Check sheet for the modelled part. Datum: model origin and axes. Units: mm. Round coordinates to 2 decimals unless told otherwise and drop trailing zeros. Write each loop counter-clockwise with the first axis right and the second up, starting at its lowest first coordinate (ties: lowest second). Pieces come first, ordered by that corner, then holes. Notation, with made-up numbers: (20.5, 0) -> (72.5, 0) arc R10 cw to (72.5, 11) -> close; hole circle Ø4 at (-14, 14.25). An arc over 180 degrees is marked (long way). One line per item, written item: value.
from build123d import *

# Parameters (mm, degrees)
F1_DEPTH         = 1
F3_W             = 38
F3_H             = 12
F4_DEPTH         = 3
F5_R             = 1.5
F7_DEPTH         = 0.7
F7_COPIES2_COUNT = 2
F9_DEPTH         = 12.5
F10_R            = 5


# Not quite as in the source:
# - a pattern or mirror of a feature is missing from the dataset's text; its kind, count and spacing are read off the source's solid


with BuildPart() as f1:
    # F0 (on Front) → F1 (new body, symmetric)
    with BuildSketch(Plane.XZ):
        with BuildLine():
            ThreePointArc((25, 31.25), (11.7164027855, 16.2518777716), (0, 0))
            Line((0, 0), (35, 0))
            ThreePointArc((35, 0), (41.1356304071, 16.2798974046), (50, 31.25))
            Line((50, 31.25), (25, 31.25))
        make_face()
        with BuildLine():
            ThreePointArc((75, 62.5), (47.6444357815, 50.6439027497), (25, 31.25))
            Line((25, 31.25), (50, 31.25))
            ThreePointArc((50, 31.25), (60.9207680237, 48.138385581), (75, 62.5))
        make_face()
    extrude(amount=F1_DEPTH, both=True)

    # F2: F1 across plane


with BuildPart() as f1_1:
    add(f1.part)
    add(f1.part.mirror(Plane.XY))

    # F3 (on Front) → F4 (join, symmetric)
    with BuildSketch(Plane.XZ):
        with Locations((-13, 0)):
            Rectangle(F3_W, F3_H)
    extrude(amount=F4_DEPTH, both=True)

    # F5
    f5_edges = [f1_1.edges().sort_by_distance(p)[0] for p in [
        (-13, 3, 6),
        (-13, -3, 6),
        (-13, -3, -6),
        (-13, 3, -6),
    ]]
    fillet(f5_edges, radius=F5_R)

    # F6 (on face) → F7 (cut)
    with BuildSketch(Plane.XZ.offset(1)):
        with BuildLine():
            Line((43.3365657685, 47.794180243), (6, 6))
            Line((6, 6), (6, 1.5))
            Line((6, 1.5), (6.0027095677, 1.5))
            Line((6.0027095677, 1.5), (52.4002239395, 53.436915958))
            ThreePointArc((52.4002239395, 53.436915958), (47.7930343948, 50.7365960242), (43.3365657685, 47.794180243))
        make_face()
        with BuildLine():
            ThreePointArc((65.9958136081, 59.6496176381), (62.8051828619, 58.40863879), (59.6589001751, 57.0591728532))
            Line((59.6589001751, 57.0591728532), (10.0254655864, 1.5))
            Line((10.0254655864, 1.5), (14.0482216051, 1.5))
            Line((14.0482216051, 1.5), (65.9958136081, 59.6496176381))
        make_face()
        with BuildLine():
            ThreePointArc((75, 62.5), (73.3655345805, 62.0514906305), (71.738905371, 61.5753443538))
            Line((71.738905371, 61.5753443538), (18.0709776237, 1.5))
            Line((18.0709776237, 1.5), (22.0937336424, 1.5))
            Line((22.0937336424, 1.5), (52.0251632611, 35.0049445138))
            ThreePointArc((52.0251632611, 35.0049445138), (62.2710885073, 49.7898624827), (75, 62.5))
        make_face()
        with BuildLine():
            Line((43.5901115949, 21.0597985398), (26.1164896611, 1.5))
            Line((26.1164896611, 1.5), (35.4331656898, 1.5))
            ThreePointArc((35.4331656898, 1.5), (38.9920250058, 11.4965917024), (43.5901115949, 21.0597985398))
        make_face()
    f7 = extrude(amount=-F7_DEPTH, mode=Mode.SUBTRACT)

    # F7_copies: F7 across plane
    add(f7.mirror(Plane.ZX), mode=Mode.SUBTRACT)

    # F7_copies1: F7 across plane
    add(f7.mirror(Plane(origin=(0, 0, 0), x_dir=(-1, 0, 0), z_dir=(0, 0, -1))), mode=Mode.SUBTRACT)

    # F7_copies2: F7 ×2 about axis
    f7_copies2_axis = Axis((0, 0, 0), (1, 0, 0))
    for i in range(1, F7_COPIES2_COUNT):
        add(f7.rotate(f7_copies2_axis, i * 360 / F7_COPIES2_COUNT), mode=Mode.SUBTRACT)

    # F8 (on face) → F9 (cut, symmetric)
    with BuildSketch(Plane.XZ.offset(1)):
        with BuildLine():
            Line((6.0027095677, 1.5), (6, 1.5))
            Line((6, 1.5), (6, -1.5))
            Line((6, -1.5), (6.0027095677, -1.5))
            Line((6.0027095677, -1.5), (10.0254655864, -1.5))
            Line((10.0254655864, -1.5), (14.0482216051, -1.5))
            Line((14.0482216051, -1.5), (18.0709776237, -1.5))
            Line((18.0709776237, -1.5), (22.0937336424, -1.5))
            Line((22.0937336424, -1.5), (26.1164896611, -1.5))
            Line((26.1164896611, -1.5), (35.4331656898, -1.5))
            ThreePointArc((35.4331656898, -1.5), (35.2136553779, -0.7508453855), (35, 0))
            ThreePointArc((35, 0), (35.2136553779, 0.7508453855), (35.4331656898, 1.5))
            Line((35.4331656898, 1.5), (26.1164896611, 1.5))
            Line((26.1164896611, 1.5), (22.0937336424, 1.5))
            Line((22.0937336424, 1.5), (18.0709776237, 1.5))
            Line((18.0709776237, 1.5), (14.0482216051, 1.5))
            Line((14.0482216051, 1.5), (10.0254655864, 1.5))
            Line((10.0254655864, 1.5), (6.0027095677, 1.5))
        make_face()
    extrude(amount=F9_DEPTH, both=True, mode=Mode.SUBTRACT)

    # F10
    f10_edges = [f1_1.edges().sort_by_distance(p)[0] for p in [
        (4.040045, 0, 6),
        (4.040045, 0, -6),
    ]]
    fillet(f10_edges, radius=F10_R)


solid = f1_1.part
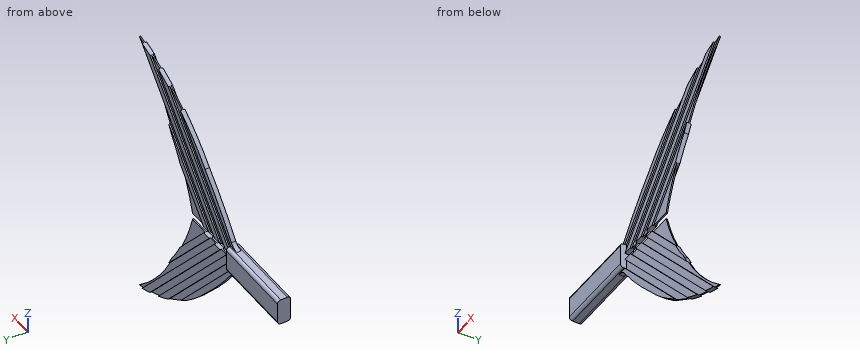
Item 1: Sectioned sample at D-D on z = 41. Enter the section's corners in (x, y), and give its area (3 significant figures).
Answer:
outline: (34.68, -1) -> (37.27, -1) -> (37.27, -0.3) -> (41.29, -0.3) -> (41.29, -1) -> (45.31, -1) -> (45.31, -0.3) -> (49.34, -0.3) -> (49.34, -1) -> (53.36, -1) -> (53.36, -0.3) -> (55.71, -0.3) -> (55.71, 0.3) -> (53.36, 0.3) -> (53.36, 1) -> (49.34, 1) -> (49.34, 0.3) -> (45.31, 0.3) -> (45.31, 1) -> (41.29, 1) -> (41.29, 0.3) -> (37.27, 0.3) -> (37.27, 1) -> (34.68, 1) -> close
area: 27.5 mm^2
Item 2: Sectioned sample at B-B on x = 67.5. Enter the section's corners in (y, z).
Answer:
outline: (-1, -60.19) -> (1, -60.19) -> (1, -56.83) -> (0.3, -56.83) -> (0.3, -55.57) -> (-0.3, -55.57) -> (-0.3, -56.83) -> (-1, -56.83) -> close; (-1, 56.83) -> (-0.3, 56.83) -> (-0.3, 55.57) -> (0.3, 55.57) -> (0.3, 56.83) -> (1, 56.83) -> (1, 60.19) -> (-1, 60.19) -> close
Item 3: Thickness scan on line 1 (Z direction, x = 17.5, y = 0.85); line 2 (X direction, y = 0.6, z = 21); line 3 (X direction, y = -0.85, z = 18). Record the ranges inside material, lowest first.
Answer:
line 1: z = -23.16 to -18.87, -14.37 to -9.87, -5.36 to -1.5, 1.5 to 5.36, 9.87 to 14.37, 18.87 to 23.16
line 2: x = 15.64 to 19.4, 23.42 to 27.45, 31.47 to 35.49, 39.51 to 43.54
line 3: x = 13.13 to 16.72, 20.74 to 24.77, 28.79 to 32.81, 36.83 to 40.86
Item 4: Depth check by flat-ended pin: P1, Ø24, axis at x = 34.5, z = -16.5, coming from the +Y side; P2, Ø0.9, axis at x = -9, y = 0, coming from the +Z side; P3, Ø0.9, axis at x = -13.5, y = 0.5, coming from the -Z side; P4, Ø6, axis at x = 3.5, z = -5.5, coming from the -Y side. Enter the tip coordinate at first touch or a pass-through.
Answer:
P1: stops at y = 1
P2: stops at z = 6
P3: stops at z = -6
P4: stops at y = -3
Item 5: Sectioned sample at A-A on x = -1.5. Enter the section's corners in (y, z).
Answer:
outline: (-3, -4.5) arc R1.5 ccw to (-1.5, -6) -> (1.5, -6) arc R1.5 ccw to (3, -4.5) -> (3, 4.5) arc R1.5 ccw to (1.5, 6) -> (-1.5, 6) arc R1.5 ccw to (-3, 4.5) -> close
